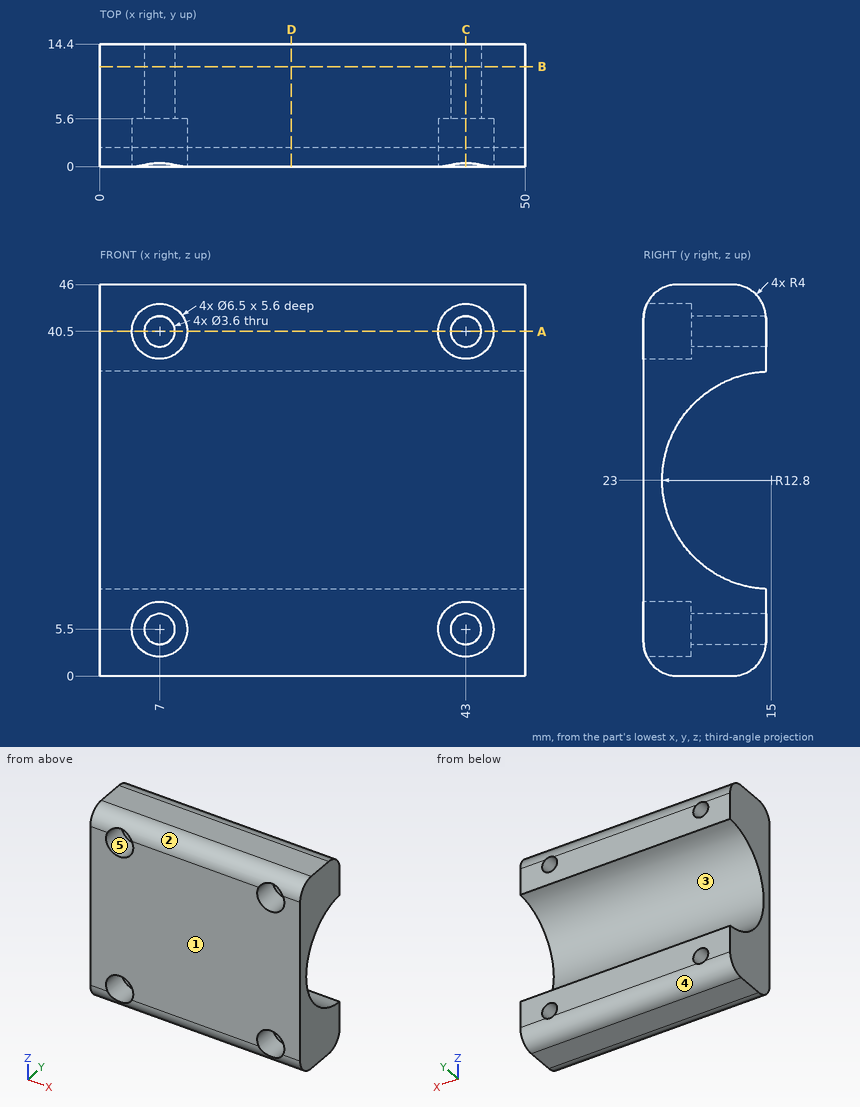
Input: dimensioned drawing with shaded views. Units: mm. Origin: part minimum x, y, z. A direction names the side the tool comes from. Coordinates: 2 decimals unless noted, no trailing zeros. Loops run counter-clockwise (first coordinate to the right, second up) from the corner with the lowest first, then second, coordinate; pieces in that order, holes last. Notation, with made-up numbers: M -40,-25.75 L -12,-25.75 A25 cw -12,8.25 Z; hole C 15,11 d6. An arc over 180 degrees is marked long. One line per item, written item: value. Start each with the question number.
1) Cut plane A-A (z = 40.5). Return loops of the section in (x, y), then the cut area to 3 significant figures.
2) Pin query (flat end, axial travel): P1, Ø3, axis at x = 7, z = 5.5, coming from the +Y side; P2, Ø2, axis at x = 8.5, z = 41.5, coming from the -Y side; P3, Ø1.5, axis at x = 43.5, y = 1.5, coming from the -Z side; P4, Ø8, axis at x = 23, z = 30, coming from the +Y side. Return the tip coordinate at first contact, or that it passes through.
3) Draft query along Z for the marked faces 1, 2 and 3. Return one class per face: released by +Z, released by -Z, zero draft, split by the parting line, or undercut.
4) Cut plane D-D (x = 22.5). Return loops of the section in (y, z), then the cut area to 3 significant figures.
5) Cut plane B-B (y = 11.75). Return loops of the section in (x, z), then the cut area to 3 significant figures.
6) Material intervals for L1, parallel to X at y = 11.75, z = 5.5; L2, parallel to X at y = 4.05, z = 5.5; L3, parallel to Z at x = 43, y = 1.55, sorted ascending. Write a range as from..to.
7) Cut plane C-C (x = 43). Return loops of the section in (y, z).
8) Reachability of the marked faces 4 and 5 from +Z, -Z, +X, -X, +Y, -Y: full face, straight path, thin tool, end or side. Return the list, or none.
Evaluation:
1. outline: M 0,0 L 3.75,0 L 3.75,5.6 L 5.2,5.6 L 5.2,14.4 L 0,14.4 Z; M 8.8,5.6 L 10.25,5.6 L 10.25,0 L 39.75,0 L 39.75,5.6 L 41.2,5.6 L 41.2,14.4 L 8.8,14.4 Z; M 44.8,5.6 L 46.25,5.6 L 46.25,0 L 50,0 L 50,14.4 L 44.8,14.4 Z
1. area: 584 mm^2
2. P1: through
2. P2: y = 5.6
2. P3: z = 0.4
2. P4: y = 8.45
3. face 1: zero draft
3. face 2: released by +Z
3. face 3: undercut
4. outline: M 0,4 A4 ccw 4,0 L 10.4,0 A4 ccw 14.4,4 L 14.4,10.21 A12.8 cw 14.4,35.79 L 14.4,42 A4 ccw 10.4,46 L 4,46 A4 ccw 0,42 Z
4. area: 407 mm^2
5. outline: M 0,0.23 L 50,0.23 L 50,10.62 L 0,10.62 Z; M 0,35.38 L 50,35.38 L 50,45.77 L 0,45.77 Z; hole C 7,5.5 d3.6; hole C 7,40.5 d3.6; hole C 43,5.5 d3.6; hole C 43,40.5 d3.6
5. area: 998 mm^2
6. L1: 0..5.2, 8.8..41.2, 44.8..50
6. L2: 0..3.75, 10.25..39.75, 46.25..50
6. L3: 0.84..2.25, 8.75..37.25, 43.75..45.16
7. outline: M 0,8.75 L 5.6,8.75 L 5.6,7.3 L 14.4,7.3 L 14.4,10.21 A12.8 cw 14.4,35.79 L 14.4,38.7 L 5.6,38.7 L 5.6,37.25 L 0,37.25 Z; M 0.4,2.25 A4 ccw 4,0 L 10.4,0 A4 ccw 14.39,3.7 L 5.6,3.7 L 5.6,2.25 Z; M 0.4,43.75 L 5.6,43.75 L 5.6,42.3 L 14.39,42.3 A4 ccw 10.4,46 L 4,46 A4 ccw Z
8. face 4: -Z, +X, -X, +Y
8. face 5: -Y
